```python
from build123d import *

# Parameters (mm, degrees)
SKETCH2_W             = 3.175
SKETCH2_H             = 9.5504
BOSS_EXTRUDE5_DEPTH   = 38.1
BOSS_EXTRUDE5_2_DEPTH = 38.1
BOSS_EXTRUDE6_DEPTH   = 3.175
SKETCH3_W             = 12.7
SKETCH3_H             = 24.700794202
BOSS_EXTRUDE7_DEPTH   = 38.1
SKETCH4_R             = 3.2258
CUT_EXTRUDE1_DEPTH    = 30.48


with BuildPart() as part:
    # Sketch2 → Boss-Extrude5 (new body)
    with BuildSketch(Plane(origin=(0, 0, 0), x_dir=(1, 0, 0), z_dir=(0, 1, 0))):
        with Locations((1.5875, 4.7752)):
            Rectangle(SKETCH2_W, SKETCH2_H)
    extrude(amount=BOSS_EXTRUDE5_DEPTH)



with BuildPart() as body_2:
    # Sketch2 → Boss-Extrude5 2 (new body)
    with BuildSketch(Plane(origin=(0, 0, 0), x_dir=(1, 0, 0), z_dir=(0, 1, 0))):
        with Locations((1.5875, 37.1348)):
            Rectangle(SKETCH2_W, SKETCH2_H)
    extrude(amount=BOSS_EXTRUDE5_2_DEPTH)


with BuildPart() as part_1:
    add(part.part)

    add(body_2.part)  # Boss-Extrude6 merges body 2
    # Sketch2<11> → Boss-Extrude6 (add)
    with BuildSketch(Plane(origin=(0, 0, 0), x_dir=(1, 0, 0), z_dir=(0, 1, 0))):
        Polygon((0, 32.3596), (0, 20.955), (0, 9.5504), (3.175, 9.5504), (3.175, 0), (101.6, 0), (101.6, 41.91), (3.175, 41.91), (3.175, 32.3596), align=None)
    extrude(amount=BOSS_EXTRUDE6_DEPTH)

    # Sketch3 → Boss-Extrude7 (add)
    with BuildSketch(Plane(origin=(0, 3.175, 0), x_dir=(1, 0, 0), z_dir=(0, 1, 0))):
        with Locations((95.25, 20.955)):
            Rectangle(SKETCH3_W, SKETCH3_H)
    extrude(amount=BOSS_EXTRUDE7_DEPTH)

    # Sketch4 → Cut-Extrude1 (cut)
    with BuildSketch(Plane.ZY.offset(-88.9)):
        with Locations((-26.150217101, 31.9024)):
            Circle(SKETCH4_R)
    extrude(amount=-CUT_EXTRUDE1_DEPTH, mode=Mode.SUBTRACT)


solid = part_1.part
```
Work out the finished part from the listing and answer in its coordinate system (mm). A direction names the side the tool comes from. Coordinates: 2 decimals unless noted, no trailing zeros. Write each loop counter-clockwise with the first axis right and the second up, starting at its lowest first coordinate (ties: lowest second). Pieces come first, ordered by that corner, then holes.
Q1. A cutting plane is placed at B-B, the plane z = -17. Give the vertices of the cut face in (x, y) (3 decimals).
Q2. Find the intervals of material crossed by line 1 (X direction, y = 18.5, z = -36) (3 decimals); line 2 (X direction, y = 39, z = -18), in increasing order.
Q3. Which of the six approach directions +Z, -Z, +X, -X, +Y, -Y give full straight-line access (tool end or side, diameter ignored) to faces 5 (the face through (95, 22, -33.305)), 6 (the face through (95, 22, -8.605)), 7 (the face through (101.6, 20, -21))?
Q4. Determine the mould class of faces 1 (the face through (2, 38.1, -37)), 2 (the face through (36, 2, 0)), 3 (the face through (2, 20, -9.55)), 4 (the face through (2, 20, -32.36)) for opening direction Z: released by +Z, released by -Z, zero draft, split by the parting line, or undercut.
Q5. A cutting plane is placed at C-C, the plane x = 78.5. Give the vertices of the cut face in (y, z) (3 decimals), then the cut area to 3 significant figures.
Q6. A cutting plane is placed at D-D, the plane z = -5. Give the vertices of the cut face in (x, y) (3 decimals).
Q7. Each of these flat-tipped pins is pushed along its axis until it touches: pin 1 Ø3.5 at (x, y) = (2.5, 17.5) entering from +Z; pin 2 Ø5 at (y, z) = (31.9, -26.15) entering from -X; pin 3 Ø7.5 at (y, z) = (13, -24) entering from -X; pin 4 Ø6.5 at (x, y) = (97.5, 29) entering from -Z. Where does it stop, or does it pass through?
Q8. A cutting plane is placed at A-A, the plane y = 12.5. Give the vertices of the cut face in (x, z) (3 decimals).
Findings below:
1. outline: (0, 0) - (101.6, 0) - (101.6, 41.275) - (88.9, 41.275) - (88.9, 3.175) - (0, 3.175) - close
2. line 1: x = 0 to 3.175
2. line 2: x = 88.9 to 101.6
3. face 5: -Z, +X, +Y
3. face 6: +Z, +X, +Y
3. face 7: +Z, -Z, +X, +Y, -Y
4. face 1: zero draft
4. face 2: released by +Z
4. face 3: undercut
4. face 4: undercut
5. outline: (0, -41.91) - (3.175, -41.91) - (3.175, 0) - (0, 0) - close
5. area: 133 mm2
6. outline: (0, 0) - (101.6, 0) - (101.6, 3.175) - (3.175, 3.175) - (3.175, 38.1) - (0, 38.1) - close
7. pin 1: stops at z = 0
7. pin 2: passes through
7. pin 3: stops at x = 88.9
7. pin 4: stops at z = -33.31
8. outline: (0, -41.91) - (3.175, -41.91) - (3.175, -32.36) - (0, -32.36) - close; (0, -9.55) - (3.175, -9.55) - (3.175, 0) - (0, 0) - close; (88.9, -33.305) - (101.6, -33.305) - (101.6, -8.605) - (88.9, -8.605) - close
